Geometry check sheet. Reference: the model listing, model coordinates, mm. Face numbers are marked on the shaded views. A direction names the side the tool comes from. Round coordinates to 2 decimals unless told otherwise and drop trailing zeros. Loops run counter-clockwise (first coordinate to the right, second up) from the corner with the lowest first, then second, coordinate; pieces in that order, holes last.
```python
from build123d import *

# Parameters (mm, degrees)
F0_R     = 12.7
F1_DEPTH = 30.1625
F2_W     = 5.08
F2_H     = 22.3266
F2_W_2   = 65.9883690595
F3_DEPTH = 254
F5_DEPTH = 19.05
F7_DEPTH = 19.05
F8_R     = 5.08


with BuildPart() as f1:
    # F0 (on Front) → F1 (new body, symmetric)
    with BuildSketch(Plane.XZ):
        with BuildLine():
            Line((108.2802, 0), (-63.5762, 0))
            ThreePointArc((-63.5762, 0), (-101.7334507731, 15.8052507731), (-85.9282, -22.352))
            Line((-85.9282, -22.352), (108.2802, -22.352))
            Line((108.2802, -22.352), (108.2802, 0))
        make_face()
        with Locations((-85.9282, 0)):
            Circle(F0_R, mode=Mode.SUBTRACT)
    extrude(amount=F1_DEPTH, both=True)

    # F2 (on face) → F3 (cut, symmetric)
    with BuildSketch(Plane.XY):
        with Locations((-61.0362, 0)):
            Rectangle(F2_W, F2_H)
        with Locations((-96.5703845298, 0)):
            Rectangle(F2_W_2, F2_H)
    extrude(amount=F3_DEPTH, both=True, mode=Mode.SUBTRACT)

    # F4 (on face) → F5 (cut)
    with BuildSketch(Plane.XZ.offset(30.1625)):
        Polygon((31.3182, 0), (-0.0762, 0), (5.9182, -22.352), (31.3182, -22.352), align=None)
    extrude(amount=-F5_DEPTH, mode=Mode.SUBTRACT)

    # F6 (on face) → F7 (join)
    with BuildSketch(Plane.XZ.offset(30.1625)):
        with BuildLine():
            ThreePointArc((64.1604, 29.718), (62.6725024484, 33.3101024484), (59.0804, 34.798))
            Line((59.0804, 34.798), (45.1104, 34.798))
            ThreePointArc((45.1104, 34.798), (41.5362153616, 16.0823576341), (31.3182, 0))
            Line((31.3182, 0), (64.1604, 0))
            Line((64.1604, 0), (64.1604, 29.718))
        make_face()
    extrude(amount=-F7_DEPTH)

    # F8
    f8_edges = [f1.edges().sort_by_distance(p)[0] for p in [
        (-63.5762, -20.6629, 0),
        (-63.5762, 20.6629, 0),
        (108.2802, 0, 0),
    ]]
    fillet(f8_edges, radius=F8_R)


solid = f1.part
```
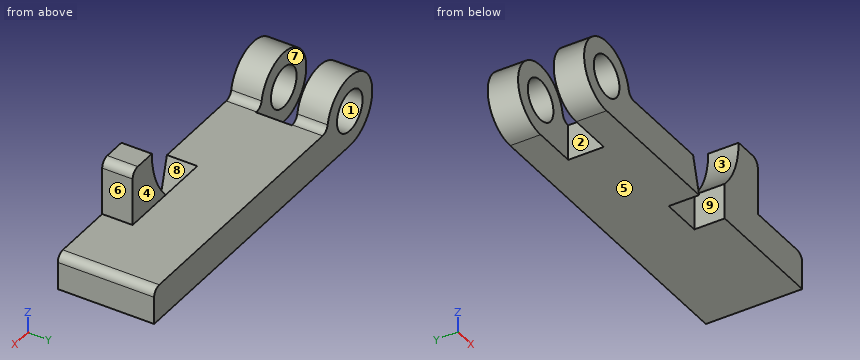
1) Mould release check, pull along X, two halves, no side actions. Record for the marked faces 1, 2, 3 and 4: +X half, -X half, draft (parallel to the pull), parting line (faces both ways), or undercut.
Report:
face 1: undercut
face 2: -X half
face 3: undercut
face 4: draft
2) Scan lines: line 1 along Y through (x, z) = (-96, 8.5); line 2 along Z through (x, y) = (-46, 24); line 3 along X through (y, z) = (-11.5, 19). Record each from-to range of solid material in increasing order.
Report:
line 1: y = -30.16 to -11.16, 11.16 to 30.16
line 2: z = -22.35 to 0
line 3: x = -97.7 to -74.15, 42.59 to 64.16
3) Gauge pin test, flat ends, axial feed: pin 1 (12 mm diameter, centred on x = 3, y = -22, fed in from +Z); pin 2 (10 mm diameter, centred on y = 23.5, z = 10, fed in from -X); pin 3 (16.5 mm diameter, centred on x = 50, z = 21, fed in from +Y); pin 4 (15 mm diameter, centred on y = -19, z = -7, fed in from -X). Record the tip position at first contact, or that the pin passes through.
Report:
pin 1: stops at z = 0
pin 2: stops at x = -107.71
pin 3: stops at y = -11.11
pin 4: stops at x = -108.28
4) Access from +Z, -Z, +X, -X, +Y, -Y to the whole of each face (thin tool, end or side, straight path). Record for the marked faces 5, 6, 7, 8 and 9.
Report:
face 5: -Z, +X, -X, +Y, -Y
face 6: +Z, +X, +Y, -Y
face 7: +Z, -Z, -X
face 8: +Z, -Y
face 9: +Z, -Z, -Y
5) Sectioned sample at B-B, the plane z = 7.5. Record the cut outline in (x, y), then the cut area to 3 significant figures.
Report:
outline: (-106.98, -30.16) - (-96.18, -30.16) - (-96.18, -11.16) - (-106.98, -11.16) - close; (-106.98, 11.16) - (-96.18, 11.16) - (-96.18, 30.16) - (-106.98, 30.16) - close; (-75.68, -30.16) - (-64.87, -30.16) - (-64.87, -11.16) - (-75.68, -11.16) - close; (-75.68, 11.16) - (-64.87, 11.16) - (-64.87, 30.16) - (-75.68, 30.16) - close; (37.15, -30.16) - (64.16, -30.16) - (64.16, -11.11) - (37.15, -11.11) - close
area: 1,340 mm2
6) Sectioned sample at C-C, the plane y = 2.5. Record the cut outline in (x, z), then the cut area to 3 significant figures.
Report:
outline: (-58.5, -22.35) - (108.28, -22.35) - (108.28, -5.08) arc R5.08 ccw to (103.2, 0) - (-58.5, 0) - close
area: 3,720 mm2
7) Sectioned sample at D-D, the plane x = -22.5. Record the cut outline in (y, z).
Report:
outline: (-30.16, -22.35) - (30.16, -22.35) - (30.16, 0) - (-30.16, 0) - close
8) Sectioned sample at A-A, the plane y = 26. Record the cut outline in (x, z).
Report:
outline: (-85.93, -22.35) - (108.28, -22.35) - (108.28, -5.08) arc R5.08 ccw to (103.2, 0) - (-58.97, 0) arc R5.08 cw to (-63.96, 4.14) arc R22.35 ccw (long way) to start; hole circle Ø25.4 at (-85.93, 0)
